from build123d import *

# Parameters (mm, degrees)
BOSS_EXTRUDE1_OUTLINE_R   = 1.600127185
BOSS_EXTRUDE1_OUTLINE_R_2 = 3.5
BOSS_EXTRUDE1_OUTLINE_R_3 = 2
BOSS_EXTRUDE1_OUTLINE_W   = 100
BOSS_EXTRUDE1_OUTLINE_H   = 42
BOSS_EXTRUDE1_DEPTH       = 1
M3_CLEARANCE_HOLE1_D      = 3.4
M3_CLEARANCE_HOLE1_DEPTH  = 4
M3_CLEARANCE_HOLE1_TIP    = 1.021463052


# Read off the part's stored shape, not the designer's step: Boss-Extrude1
with BuildPart() as part:
    # Boss-Extrude1 outline → Boss-Extrude1 (new body)
    with BuildSketch(Plane.XY):
        with BuildLine():
            ThreePointArc((110.511379674, -48.456994218), (111.925593237, -47.871207781), (112.511379674, -46.456994218))
            Line((112.511379674, -46.456994218), (112.511379674, 47.163183245))
            ThreePointArc((112.511379674, 47.163183245), (111.925593236, 48.577396807), (110.511379674, 49.163183245))
            Line((110.511379674, 49.163183245), (-14.651641589, 49.163183245))
            ThreePointArc((-14.651641589, 49.163183245), (-16.065855151, 48.577396807), (-16.651641589, 47.163183245))
            Line((-16.651641589, 47.163183245), (-16.651641589, -46.456994218))
            ThreePointArc((-16.651641589, -46.456994218), (-16.065855152, -47.871207781), (-14.651641589, -48.456994218))
            Line((-14.651641589, -48.456994218), (110.511379674, -48.456994218))
        make_face()
        with BuildLine():
            Line((4.864408455, -22.627663705), (4.864408455, -32.627663705))
            ThreePointArc((4.864408455, -32.627663705), (2.364408455, -35.127663705), (-0.135591545, -32.627663705))
            Line((-0.135591545, -32.627663705), (-0.135591545, -22.627663705))
            ThreePointArc((-0.135591545, -22.627663705), (2.364408455, -20.127663705), (4.864408455, -22.627663705))
        make_face(mode=Mode.SUBTRACT)
        with Locations((1.954046296, -15.88396989)):
            Circle(BOSS_EXTRUDE1_OUTLINE_R, mode=Mode.SUBTRACT)
        with Locations((48.457742604, -27.384884031)):
            Circle(BOSS_EXTRUDE1_OUTLINE_R_2, mode=Mode.SUBTRACT)
        with Locations((88.460922224, -27.384884031)):
            Circle(BOSS_EXTRUDE1_OUTLINE_R_3, mode=Mode.SUBTRACT)
        with Locations((94.961438913, -15.88396989)):
            Circle(BOSS_EXTRUDE1_OUTLINE_R, mode=Mode.SUBTRACT)
        with Locations((1.954046296, 39.120402088)):
            Circle(BOSS_EXTRUDE1_OUTLINE_R, mode=Mode.SUBTRACT)
        with Locations((48.454046296, 11.620402088)):
            Rectangle(BOSS_EXTRUDE1_OUTLINE_W, BOSS_EXTRUDE1_OUTLINE_H, mode=Mode.SUBTRACT)
        with Locations((94.961438913, 39.120402088)):
            Circle(BOSS_EXTRUDE1_OUTLINE_R, mode=Mode.SUBTRACT)
    extrude(amount=BOSS_EXTRUDE1_DEPTH)

    # M3 Clearance Hole1
    with Locations(Plane.XY.offset(1)):
        with Locations((-11.651641589, 44.163183245), (-11.651641589, -43.456994218), (107.511379674, -43.456994218), (107.511379674, 44.163183245), (34.949251299, -43.456994218), (60.929869042, -43.456994218)):
            Hole(M3_CLEARANCE_HOLE1_D / 2, depth=M3_CLEARANCE_HOLE1_DEPTH)
            with Locations((0, 0, -(M3_CLEARANCE_HOLE1_DEPTH + M3_CLEARANCE_HOLE1_TIP / 2))):  # 118° drill point
                Cone(0, M3_CLEARANCE_HOLE1_D / 2, M3_CLEARANCE_HOLE1_TIP, mode=Mode.SUBTRACT)


solid = part.part
Here's how the part is built. I have some questions about the finished solid (model axes, mm). A direction names the side the tool comes from. Round coordinates to 2 decimals unless told otherwise and drop trailing zeros. Loops run counter-clockwise (first coordinate to the right, second up) from the corner with the lowest first, then second, coordinate; pieces in that order, holes last. Notation, with made-up numbers: (-17, 18) - (27, 18) arc R22 cw to (27, 48) - close; hole circle Ø9 at (56, -10.5). An arc over 180 degrees is marked (long way). One line per question, with ' | ' between items. Start each with the question number.
Q1. I want a section at B-B (y = 10). Write out the boundary of the cut face in (x, z).
Q2. Please list where these lines run through material, in increasing order: line 1 (Y direction, x = 48, z = 0.2); line 2 (X direction, y = -27.5, z = 0.2); line 3 (X direction, y = -6.5, z = 0.4). Write a range as [from, to].
Q3. I want a section at D-D (z = 0.15). State how many separate pieces and enclosed holes the cut face has, then the cut area to 3 significant figures.
Q4. We'd pull the mould along Y, two halves only. Please class faces 3 (the cylindrical face through (45.68, -29.515, 0.493)), 4 (the flat face through (47, -10, 0)): +Y half, -Y half, draft (parallel to the pull), parting line (faces both ways), or undercut.
Q5. For faces 1 (the cylindrical face through (2.419, -35.127, 0.493)), 2 (the flat face through (47, -10, 1)), which set-ups out of +Z, -Z, +X, -X, +Y, -Y let a thin tool reach every point of the face, with its end or its side?
Q6. I want a section at A-A (x = 76). Write out the boundary of the cut face in (y, z).
Q7. Will this pin go through, and if not, where does the flat tip stop? pin 1 (2.5 mm diameter, centred on x = 94.96, y = 39.12, fed in from +Z).
Q8. I want a section at C-C (x = 50). Write out the boundary of the cut face in (y, z), then the cut area to 3 significant figures.
Response values:
1) outline: (-16.65, 0) - (-1.55, 0) - (-1.55, 1) - (-16.65, 1) - close; (98.45, 0) - (112.51, 0) - (112.51, 1) - (98.45, 1) - close
2) line 1: y = [-48.46, -30.85], [-23.91, -9.38], [32.62, 49.16] | line 2: x = [-16.65, -0.14], [4.86, 44.96], [51.96, 86.46], [90.46, 112.51] | line 3: x = [-16.65, -1.55], [98.45, 112.51]
3) separate pieces: 1 | enclosed holes: 14 | area: 8,200 mm²
4) face 3: undercut | face 4: draft
5) face 1: +Z, -Z | face 2: +Z, +X, -X, +Y, -Y
6) outline: (-48.46, 0) - (-9.38, 0) - (-9.38, 1) - (-48.46, 1) - close; (32.62, 0) - (49.16, 0) - (49.16, 1) - (32.62, 1) - close
7) pin 1: passes through
8) outline: (-48.46, 0) - (-30.53, 0) - (-30.53, 1) - (-48.46, 1) - close; (-24.24, 0) - (-9.38, 0) - (-9.38, 1) - (-24.24, 1) - close; (32.62, 0) - (49.16, 0) - (49.16, 1) - (32.62, 1) - close | area: 49.3 mm²
